Print and shaded views of the part. All mm, measured from the part's lowest x, y and z. A direction names the side the tool comes from. Coordinates: 2 decimals unless noted, no trailing zeros. Loops run counter-clockwise (first coordinate to the right, second up) from the corner with the lowest first, then second, coordinate; pieces in that order, holes last. Notation, with made-up numbers: M -24,50 L 11,50 A17 cw 11,57 Z; hole C -24,-24.5 d10. An arc over 180 degrees is marked long. Answer as a JSON object with one key per item and string values. Group by question number.
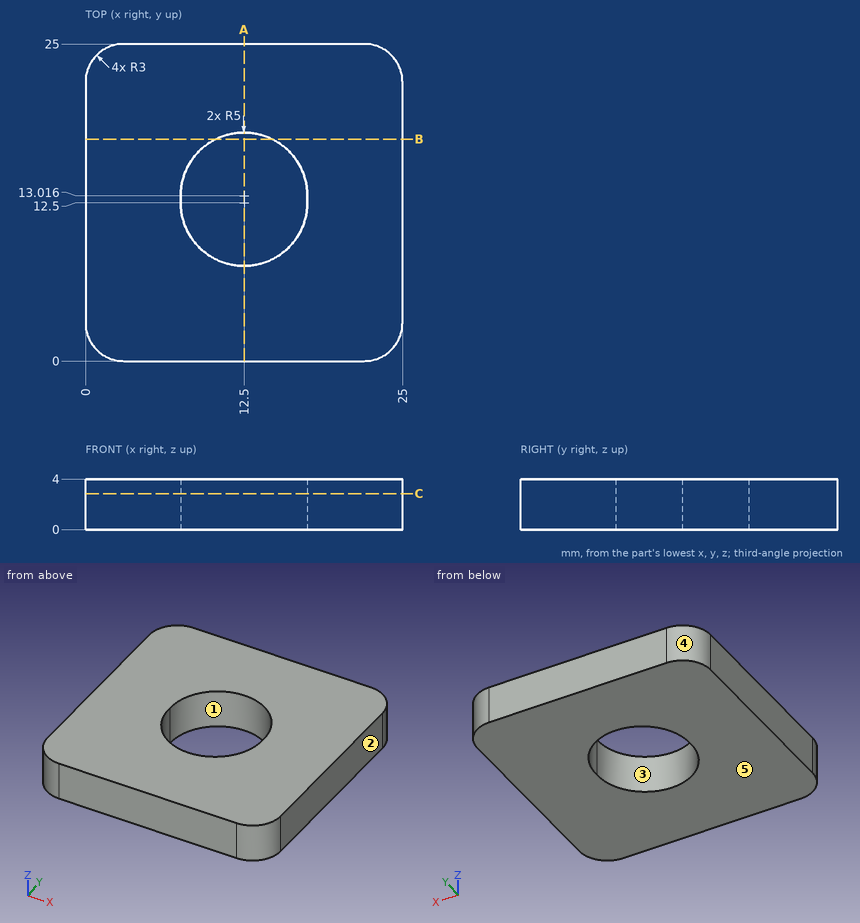
Item 1: Slice it at B-B, the plane y = 17.5. Write the cut outline in (x, z).
Item 2: Tool access for the marked faces 1 and 2: list every direction of +Z, -Z, +X, -X, +Y, -Y with a clear straight run to the whole face (end or side of a thin tool).
Item 3: Drill centre lines: L1, parallel to X at y = 13.25, z = 3.5 (1 decimal); L2, parallel to Y at x = 10.25, z = 2.55 (1 decimal); L3, parallel to X at y = 15.75, z = 3.45 (1 decimal). Where is each one in solid material? Low to high. Write a range as from..to.
Item 4: Pull direction X, two halves, no side cores. Call the marked faces 3, 4 and 5: released by +X, released by -X, zero draft, split by the parting line, or undercut.
Item 5: Slice it at C-C, the plane z = 2.85. Write the cut outline in (x, y).
Item 6: Slice it at A-A, the plane x = 12.5. Write the cut outline in (y, z).
Computed:
{
 "1": {"outline": "M 0,0 L 10.29,0 L 10.29,4 L 0,4 Z; M 14.71,0 L 25,0 L 25,4 L 14.71,4 Z"},
 "2": {"face 1": "+Z, -Z", "face 2": "+Z, -Z, +X, +Y, -Y"},
 "3": {"L1": "0..7.5, 17.5..25", "L2": "0..8, 17.5..25", "L3": "0..8.3, 16.7..25"},
 "4": {"face 3": "undercut", "face 4": "released by -X", "face 5": "zero draft"},
 "5": {"outline": "M 0,3 A3 ccw 3,0 L 22,0 A3 ccw 25,3 L 25,22 A3 ccw 22,25 L 3,25 A3 ccw 0,22 Z; hole M 7.51,12.76 A5 ccw long 17.49,12.76 A5 ccw long Z"},
 "6": {"outline": "M 0,0 L 7.5,0 L 7.5,4 L 0,4 Z; M 18.02,0 L 25,0 L 25,4 L 18.02,4 Z"}
}
